from build123d import *

# Parameters (mm, degrees)
SKETCH_2_R          = 5
CUT_EXTRUDE_1_DEPTH = 20
SKETCH_3_R          = 9
CUT_EXTRUDE_2_DEPTH = 5


with BuildPart() as part:
    # Эскиз1 → Повернуть1 (revolve)
    with BuildSketch(Plane.XY, mode=Mode.PRIVATE) as revolve_1_sk:
        Polygon((0, 0), (100, 0), (100, 15), (40, 15), (40, 35), (10, 35), (10, 20), (0, 20), align=None)
    revolve(revolve_1_sk.sketch.rotate(Axis((0, 0, 0), (1, 0, 0)), 90), axis=Axis((0, 0, 0), (1, 0, 0)))

    # Эскиз2 → Вырез-Вытянуть1 (cut)
    with BuildSketch(Plane(origin=(0, 0, 0), x_dir=(0, 0, -1), z_dir=(1, 0, 0))):
        Circle(SKETCH_2_R)
    extrude(amount=CUT_EXTRUDE_1_DEPTH, mode=Mode.SUBTRACT)

    # Эскиз3 → Вырез-Вытянуть2 (cut)
    with BuildSketch(Plane(origin=(0, 0, 0), x_dir=(0, 0, -1), z_dir=(1, 0, 0))):
        Circle(SKETCH_3_R)
    extrude(amount=CUT_EXTRUDE_2_DEPTH, mode=Mode.SUBTRACT)


solid = part.part
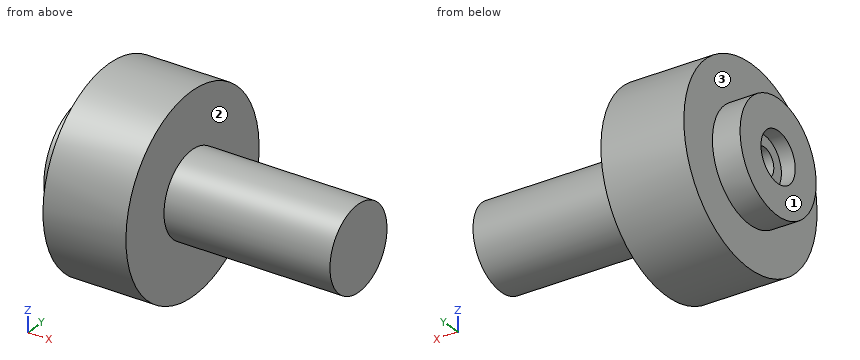
Part model, mm, in its own coordinate system. Face numbers are marked on the shaded views. A direction names the side the tool comes from. Give positions to 0.01 mm unless a question says otherwise; leave off trailing zeros. Order: outer loops, then holes, each group sorted by start corner. A loop starts at its lowest first (then second) coordinate and runs counter-clockwise, first axis right, second up. Notation, with made-up numbers: (85, -37.5) -> (136, -37.5) arc R16 cw to (136, -7.5) -> close; hole circle Ø7 at (20.5, 22.5). An arc over 180 degrees is marked (long way). Use one line per item in the form item = value.
(1) Saw through at A-A (z = 0). Write the cut outline in (x, y).
Solution:
outline = (0, -20) -> (10, -20) -> (10, -35) -> (40, -35) -> (40, -15) -> (100, -15) -> (100, 15) -> (40, 15) -> (40, 35) -> (10, 35) -> (10, 20) -> (0, 20) -> (0, 9) -> (5, 9) -> (5, 5) -> (20, 5) -> (20, -5) -> (5, -5) -> (5, -9) -> (0, -9) -> close
(2) Tool access for the marked faces 1, 2 and 3: list every direction of +Z, -Z, +X, -X, +Y, -Y with a clear straight run to the whole face (end or side of a thin tool).
Solution:
face_1 = +Z, -Z, -X, +Y, -Y
face_2 = +X
face_3 = -X
(3) Saw through at D-D (x = 65). Write the cut outline in (y, z).
Solution:
outline = circle Ø30 at (0, 0)
(4) Drill centre lines: line 1 (Y direction, x = 3, z = 0); line 2 (Y direction, x = 11.5, z = 0); line 3 (X direction, y = -13.5, z = 21.5). Where is each one in solid material? Low to high. Write a range as from..to.
Solution:
line_1 = -20..-9, 9..20
line_2 = -35..-5, 5..35
line_3 = 10..40
(5) Flat gauge pins, fed straight in: P1, Ø8, axis at y = 0.5, z = -1, coming from the -X side; P2, Ø10, axis at x = 70.5, z = 4.5, coming from the +Y side; P3, Ø1, axis at x = 25.5, y = -4, coming from the -Z side. Where does each tip first touch, or does it go through?
Solution:
P1 = 5
P2 = 15
P3 = -34.82
(6) Saw through at B-B (x = 18.5). Write the cut outline in (y, z).
Solution:
outline = circle Ø70 at (0, 0); hole circle Ø10 at (0, 0)
